Geometry check sheet. Reference: drawing and pictorial views, mm from the part's lowest x, y, z. Give positions to 0.01 mm unless a question says otherwise; leave off trailing zeros. Write each loop counter-clockwise with the first axis right and the second up, starting at its lowest first coordinate (ties: lowest second). Pieces come first, ordered by that corner, then holes. Notation, with made-up numbers: (12.5, 89) -> (20.5, 89) arc R13 ccw to (20.5, 112) -> close; hole circle Ø4 at (63.25, 73). An arc over 180 degrees is marked (long way). Answer as CSV lines item,"result".
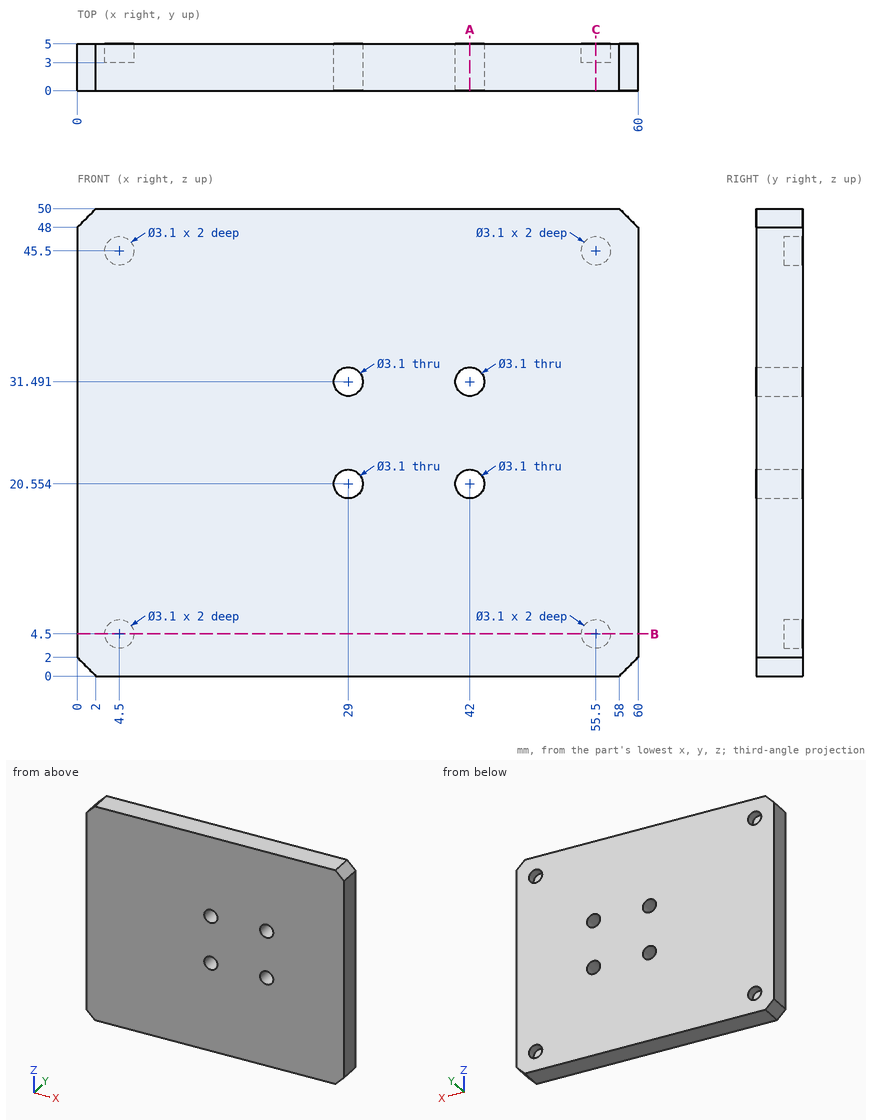
1) Section check B-B (z = 4.5). Record the boundary of the cut face in (x, y), and give its area (3 significant figures).
Reported:
outline,"(0, 0) -> (60, 0) -> (60, 5) -> (57.05, 5) -> (57.05, 3) -> (53.95, 3) -> (53.95, 5) -> (6.05, 5) -> (6.05, 3) -> (2.95, 3) -> (2.95, 5) -> (0, 5) -> close"
area,"288 mm²"
2) Scan lines: line 1 along Z through (x, y) = (29, 0.2); line 2 along X through (y, z) = (4.05, 4.5); line 3 along Z through (x, y) = (55.5, 4.5). Record each from-to range of solid material in increasing order.
Reported:
line 1,"0 to 19, 22.1 to 29.94, 33.04 to 50"
line 2,"0 to 2.95, 6.05 to 53.95, 57.05 to 60"
line 3,"0 to 2.95, 6.05 to 43.95, 47.05 to 50"
3) Section check C-C (x = 55.5). Record the boundary of the cut face in (y, z), and give its area (3 significant figures).
Reported:
outline,"(0, 0) -> (5, 0) -> (5, 2.95) -> (3, 2.95) -> (3, 6.05) -> (5, 6.05) -> (5, 43.95) -> (3, 43.95) -> (3, 47.05) -> (5, 47.05) -> (5, 50) -> (0, 50) -> close"
area,"238 mm²"
4) Section check A-A (x = 42). Record the boundary of the cut face in (y, z), and give its area (3 significant figures).
Reported:
outline,"(0, 0) -> (5, 0) -> (5, 19) -> (0, 19) -> close; (0, 22.1) -> (5, 22.1) -> (5, 29.94) -> (0, 29.94) -> close; (0, 33.04) -> (5, 33.04) -> (5, 50) -> (0, 50) -> close"
area,"219 mm²"
5) Depth check by flat-ended pin: pin 1 (3 mm diameter, centred on x = 55.5, z = 45.5, fed in from -Y); pin 2 (1.5 mm diameter, centred on x = 55.5, z = 45.5, fed in from +Y). Enter the tip coordinate at first touch or a pass-through.
Reported:
pin 1,"y = 0"
pin 2,"y = 3"
